Read the model definition and answer for the solid it produces. Units are mm, in the model's axes. Coordinates: 2 decimals unless noted, no trailing zeros. Loops run counter-clockwise (first coordinate to the right, second up) from the corner with the lowest first, then second, coordinate; pieces in that order, holes last. Notation, with made-up numbers: (77.5, -36.5) - (98.5, -36.5) arc R25 cw to (98.5, -7.5) - close; hole circle Ø4 at (32.25, -1). An arc over 180 degrees is marked (long way). Use one line per item in the form item = value.
Autodesk Inventor part; units mm, degrees
ref_plane "YZ Plane" through (0, 0, 0) normal (1, 0, 0) x (0, 1, 0)
ref_plane "XZ Plane" through (0, 0, 0) normal (0, 1, 0) x (-1, 0, 0)
ref_plane "XY Plane" through (0, 0, 0) normal (0, 0, 1) x (1, 0, 0)
sketch "スケッチ1" plane through (0, 0, 0) normal (1, 0, 0) x (0, 1, 0)
  line L0 (-78.1013, 9.4232) -> (-98.1013, 9.4232)
  line L1 (-98.1013, 9.4232) -> (-78.1013, 9.4232)
  line L2 (-78.1013, 9.4232) -> (-78.1013, -630.5768)
  line L3 (-78.1013, -630.5768) -> (-98.1013, -630.5768)
  line L4 (-98.1013, -630.5768) -> (-98.1013, 9.4232)
  line L5 (90.8987, -620.5768) -> (110.8987, -620.5768)
  line L6 (110.8987, -620.5768) -> (110.8987, -53.5768)
  line L7 (110.8987, -53.5768) -> (90.8987, -53.5768)
  line L8 (90.8987, -53.5768) -> (90.8987, -620.5768)
  line L9 (90.8987, 19.4232) -> (90.8987, 586.4232)
  line L10 (-73.5639, 640.5027) -> (90.8987, -49.1588)
  line L11 (90.8987, -49.1588) -> (110.3532, -44.5196)
  line L12 (110.3532, -44.5196) -> (-54.1094, 645.142)
  line L13 (-54.1094, 645.142) -> (-73.5639, 640.5027)
  line L14 (-78.1013, 644.9232) -> (-78.1013, 9.4232)
  circle A0 centre (-88.1013, 639.9232) radius 1.5
  circle A1 centre (-88.1013, 639.9232) radius 1.5
  circle A2 centre (-88.1013, 629.9232) radius 1.5
  circle A3 centre (-88.1013, 629.9232) radius 1.5
  line L15 (-98.1013, 9.4232) -> (-98.1013, 644.9232)
  line L16 (-98.1013, 624.9232) -> (-78.1013, 624.9232)
  line L17 (-78.1013, 624.9232) -> (-67.7648, 616.1846)
  line L18 (-67.7648, 616.1846) -> (-48.3103, 620.8239)
  line L19 (-78.1013, 644.9232) -> (-54.1094, 645.142)
  circle A4 centre (-61.517, 633.0951) radius 1.5
  circle A5 centre (-59.1973, 623.3679) radius 1.5
  line L20 (-78.1013, 644.9232) -> (-98.1013, 644.9232)
  line L21 (-78.1013, 644.9232) -> (-98.1013, 644.9232)
  line L22 (-98.1013, 644.9232) -> (-98.1013, 624.9232)
  line L23 (-98.1013, -20.5768) -> (-78.1013, -20.5768)
  circle A6 centre (-88.1013, -15.5768) radius 1.5
  line L24 (-98.1013, 39.4232) -> (-78.1013, 39.4232)
  circle A7 centre (-88.1013, 34.4232) radius 1.5
  line L25 (-98.1013, 39.4232) -> (-98.1013, 8.2286)
  line L26 (-78.1013, 39.4232) -> (-78.1013, 9.4232)
  point P0 (0, 0)
  point P1 (-78.1013, 19.4232)
  point P2 (-88.1013, -605.5768)
  point P3 (100.8987, -605.5768)
  point P4 (100.8987, -58.5768)
  point P5 (100.8987, -68.5768)
  point P6 (100.8987, -620.5768)
  point P7 (98.3063, -37.112)
  point P8 (95.9867, -27.3847)
  point P9 (-58.0375, 618.5042)
  dimension "d0" = 20
  dimension "d1" = 640
  dimension "d2" = 20
  dimension "d3" = 567
  dimension "d4" = 10
  dimension "d5" = 0
  dimension "d6" = 25
  dimension "d7" = 15
  dimension "d8" = 10
  dimension "d9" = 10
  dimension "d10" = 5
  dimension "d11" = 10
  dimension "d12" = 10
  dimension "d13" = 10
  dimension "d14" = 20
  dimension "d15" = 709
  dimension "d16" = 4.4179
  dimension "d17" = 4.5374
  dimension "d18" = 10
  dimension "d19" = 10
  dimension "d20" = 10
  dimension "d21" = 10
  dimension "d22" = 10
  dimension "d23" = 10
  dimension "d24" = 10
  dimension "d25" = 10
  dimension "d26" = 25
  dimension "d27" = 10
  dimension "d28" = 3
  dimension "d29" = 3
  dimension "d30" = 5
  dimension "d31" = 5
  dimension "d32" = 3
  dimension "d33" = 3
  dimension "d34" = 5
  dimension "d35" = 3
  dimension "d36" = 5
extrude "押し出し1" add sketch "スケッチ1" against normal blind 2 contours L2 L23 L4 L0 | L0 L15 L24 L14
fillet "フィレット1" radius 2 4 edges at (-1, -78.1013, 39.4232) (-1, -98.1013, 39.4232) (-1, -98.1013, -20.5768) (-1, -78.1013, -20.5768)
properties part number "base_weel-v1-Plate-expand-1" material "アルミニウム 6061"
Item 1: For a pull along Z with two mould halves and no side action, classify faces 1 (the cylindrical face through (-1, -89.6, 34.5)), 2 (the flat face through (-1, -78.101, 10)), 3 (the cylindrical face through (-1, -89.6, -15.5)), 4 (the cylindrical face through (-1.014, -97.5, -20.006)) as +Z half, -Z half, draft (parallel to the pull), parting line (faces both ways), or undercut.
Results below:
face_1 = undercut
face_2 = draft
face_3 = undercut
face_4 = -Z half
Item 2: Find the intervals of material crossed by L1, parallel to Z at x = -1.7, y = -88.25; L2, parallel to Y at x = -0.2, z = -16; L3, parallel to Z at x = -0.95, y = -96.75, in increasing order.
Results below:
L1 = -20.58 to -17.07, -14.08 to 32.93, 35.92 to 39.42
L2 = -98.1 to -89.54, -86.66 to -78.1
L3 = -20.47 to 39.32
Item 3: The part is cut by section A-A on y = -88.25. Give the vertices of the cut face in (x, z), plus the area to 3 significant figures.
Results below:
outline = (-2, -20.58) - (0, -20.58) - (0, -17.07) - (-2, -17.07) - close; (-2, -14.08) - (0, -14.08) - (0, 32.93) - (-2, 32.93) - close; (-2, 35.92) - (0, 35.92) - (0, 39.42) - (-2, 39.42) - close
area = 108 mm²
